from build123d import *

# Parameters (mm, degrees)
SKETCH1_W = 22
SKETCH1_H = 1


with BuildPart() as part:
    # Sweep1: sweep along a path in Sketch2
    with BuildLine(Plane(origin=(0, 0, 0), x_dir=(0, 0, -1), z_dir=(1, 0, 0))) as sweep1_path:
        Line((0, 15.5), (-27, 15.5))
        ThreePointArc((-27, 15.5), (-28.767766953, 14.767766953), (-29.5, 13))
        Line((-29.5, 13), (-29.5, -13))
        ThreePointArc((-29.5, -13), (-28.767766953, -14.767766953), (-27, -15.5))
        Line((-27, -15.5), (0, -15.5))
    # Sketch1 → Sweep1 (sweep)
    with BuildSketch(Plane.XY):
        with Locations((0, 15.5)):
            Rectangle(SKETCH1_W, SKETCH1_H)
    sweep(path=sweep1_path.line)


solid = part.part
Can you work these out from the model? Positions are in its coordinate system, mm. A direction names the side the tool comes from. Coordinates: 2 decimals unless noted, no trailing zeros. Loops run counter-clockwise (first coordinate to the right, second up) from the corner with the lowest first, then second, coordinate; pieces in that order, holes last. Notation, with made-up numbers: M 38.25,-15 L 84.25,-15 A32 ccw 84.25,18 Z; hole C 10.5,76.25 d6. An arc over 180 degrees is marked long. Return JSON: item names as keys, results as strings. Group by question number.
Item 1: If I drill on L1, parallel to Y at x = 2, z = 8.5; L2, parallel to Z at x = -9, y = 11.5; L3, parallel to Z at x = 8.25, y = 15.5, over which ranges is the centre line in solid material (lowest first)? Write a range as from..to.
Item 2: Imagine slicing it at B-B (x = 3.5). Please give me the cut outline in (y, z), and give its area (3 significant figures).
Item 3: Imagine slicing it at A-A (z = 3.5). Please give me the cut outline in (x, y), and give its area (3 significant figures).
Item 4: On a 3-axis mill with a long thin cutter (end or side, diameter ignored), from which of +Z, -Z, +X, -X, +Y, -Y can I reach the whole of each face in a straight line? I mean faces 1 (the flat face through (0, 0, 29)), 2 (the cylindrical face through (-0.15, 15.14, 29.1)). Say none if no direction works.
Item 5: Imagine slicing it at D-D (y = -14). Please give me the cut outline in (x, z).
Item 6: I'm going to push a flat-ended pin straight in: pin 1 Ø6.5 at (x, y) = (3, 5) entering from -Z. Where does the tip first touch, or does it pass through?
Item 7: Imagine slicing it at C-C (y = 6). Please give me the cut outline in (x, z).
Item 8: Thinking about a two-plate mould opening in Y: for faces 3 (the flat face through (0, 16, 14)), 4 (the flat face through (0, -15, 13)), 5 (the flat face through (-0.2, 15.5, 0)), 6 (the flat face through (0, -16, 13)), which applies, released by +Y, released by -Y, zero draft, split by the parting line, or undercut?
Verdict:
{
 "1": {"L1": "y = -16..-15, 15..16", "L2": "z = 29..30", "L3": "z = 0..28.66"},
 "2": {"outline": "M -16,0 L -15,0 L -15,27 A2 cw -13,29 L 13,29 A2 cw 15,27 L 15,0 L 16,0 L 16,27 A3 ccw 13,30 L -13,30 A3 ccw -16,27 Z", "area": "87.9 mm^2"},
 "3": {"outline": "M -11,-16 L 11,-16 L 11,-15 L -11,-15 Z; M -11,15 L 11,15 L 11,16 L -11,16 Z", "area": "44.0 mm^2"},
 "4": {"face 1": "-Z, +X, -X", "face 2": "+Z, +X, -X, +Y"},
 "5": {"outline": "M -11,28.73 L 11,28.73 L 11,29.83 L -11,29.83 Z"},
 "6": {"pin 1": "stops at z = 29"},
 "7": {"outline": "M -11,29 L 11,29 L 11,30 L -11,30 Z"},
 "8": {"face 3": "released by +Y", "face 4": "undercut", "face 5": "zero draft", "face 6": "released by -Y"}
}
